from build123d import *

# Parameters (mm, degrees)
BOSS_EXTRUDE1_DEPTH = 3.175
SKETCH2_R           = 14.2875
CUT_EXTRUDE1_DEPTH  = 837.34562622


with BuildPart() as part:
    # Sketch1 → Boss-Extrude1 (new body)
    with BuildSketch(Plane(origin=(1.950344864, 0, -26.264644174), x_dir=(-0.9972542674746705, 0, -0.07405353471346578), z_dir=(0.07405353471346578, 0, -0.9972542674746705))):
        Polygon((-183.644373355, -298.45), (-183.644373355, 298.45), (-826.760197391, 177.8), (-826.760197391, -177.8), align=None)
    extrude(amount=BOSS_EXTRUDE1_DEPTH)

    # Sketch2 → Cut-Extrude1 (cut, through all)
    with BuildSketch(Plane(origin=(825.5, 212.942802273, 150.983020837), x_dir=(1, 0, 0), z_dir=(0, 0.32191156150474026, 0.9467697431633416))):
        Circle(SKETCH2_R)
    cut_extrude1 = extrude(amount=-CUT_EXTRUDE1_DEPTH, mode=Mode.SUBTRACT)

    # Mirror1: Cut-Extrude1 across plane
    add(cut_extrude1.mirror(Plane.ZX), mode=Mode.SUBTRACT)


solid = part.part
Could you check a few things on this model? Use its own coordinates, in mm. Give positions to 0.01 mm unless a question says otherwise; leave off trailing zeros. Loops run counter-clockwise (first coordinate to the right, second up) from the corner with the lowest first, then second, coordinate; pieces in that order, holes last. Notation, with made-up numbers: (56.25, 89) -> (94.25, 89) arc R14 ccw to (94.25, 112) -> close; hole circle Ø3 at (-22.75, 70.5). An arc over 180 degrees is marked (long way). Answer as CSV lines item,"result". Start each with the question number.
(1) I'm going to push flat-ended pins straight in: pin 1 Ø8 at (x, y) = (317, 22.5) entering from -Z; pin 2 Ø4 at (x, z) = (450.5, 5) entering from -Y; pin 3 Ø6 at (x, y) = (536.5, -13.5) entering from -Z. Where does each tip first touch, or does it pass through?
(2) We'd pull the mould along Y, two halves only. Please class faces 1 (the flat face through (510.25, 4.18, 11.48)), 2 (the cylindrical face through (813.205, -164.99, 32.555)): released by +Y, released by -Y, zero draft, split by the parting line, or undercut.
(3) If we section it at A-A on y = -99: Write out the boundary of the cut face in (x, z), then the cut area to 3 significant figures.
(4) If we section it at B-B on x = 699: Write out the boundary of the cut face in (y, z), then the cut area to 3 significant figures.
(5) I need wall thicknesses on probe 1 along Z at (x, y) = (302.5, -173.5); probe 2 along Z at (x, y) = (617, 55.5); probe 3 along Y at (x, z) = (373.5, 0.5). Which ranges of each line are inside material? Lowest first, please.
Computed:
1,pin 1,"stops at z = -6.35"
1,pin 2,"stops at y = -248.93"
1,pin 3,"stops at z = 10.02"
2,face 1,"zero draft"
2,face 2,"undercut"
3,outline,"(185.09, -12.67) -> (185.33, -15.83) -> (826.68, 31.79) -> (826.44, 34.96) -> close"
3,area,"2,040 mm2"
4,outline,"(-201.82, 22.31) -> (201.82, 22.31) -> (201.77, 25.5) -> (-201.77, 25.5) -> close"
4,area,"1,280 mm2"
5,probe 1,"z = -7.13 to -3.95"
5,probe 2,"z = 16.22 to 19.41"
5,probe 3,"y = -263.02 to 263.02"
